Geometry: see drawing. Coordinates: mm, zero at the bounding-box minimum. Give positions to 0.01 mm unless a question says otherwise; leave off trailing zeros. Write each loop counter-clockwise with the first axis right and the second up, starting at its lowest first coordinate (ties: lowest second). Pieces come first, ordered by that corner, then holes. Notation, with made-up numbers: (49.25, 72.5) -> (95.25, 72.5) arc R24 cw to (95.25, 95.5) -> close; hole circle Ø1 at (-5.75, 73.5). An arc over 180 degrees is marked (long way). Answer as a JSON object with one key per item and string values. Group by question number.
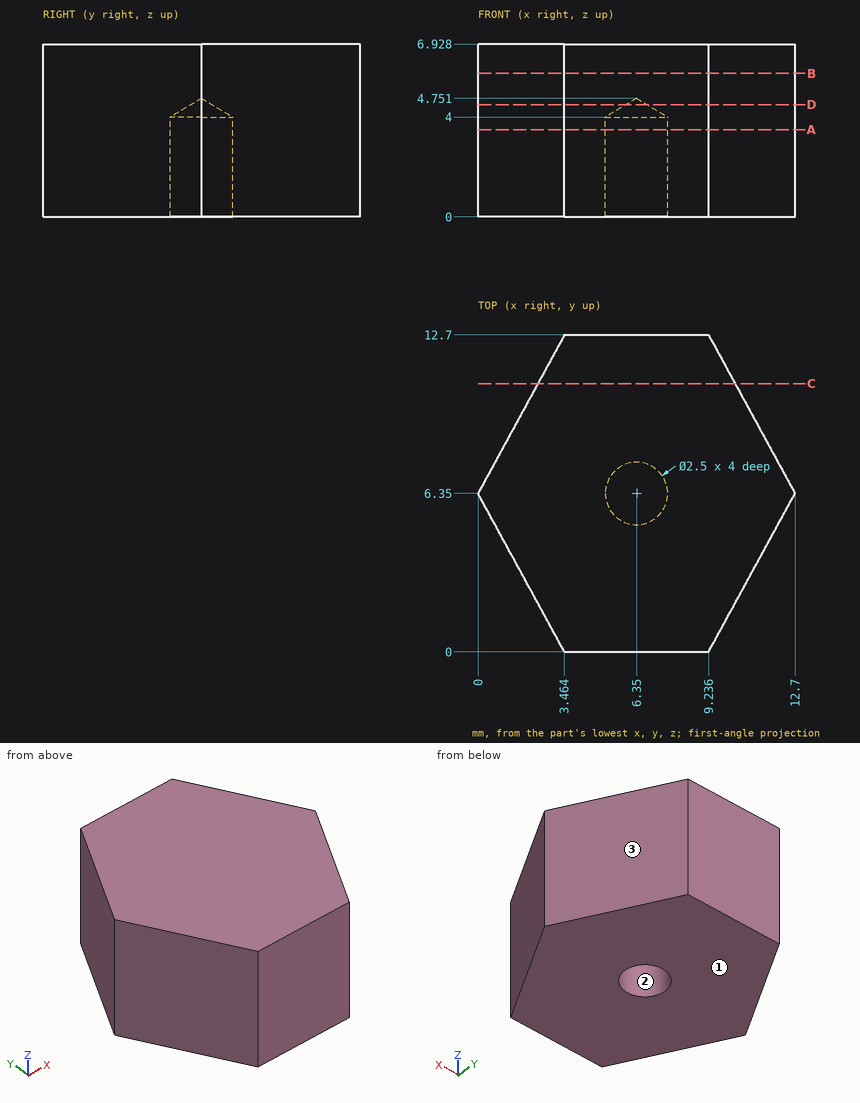
1. Section D-D (z = 4.5). Return the cut outline in (x, y), plus the area to 3 significant figures.
2. Line query: line 1 (Y direction, x = 6.35, z = 3.2); line 2 (Y direction, x = 5.75, z = 2); line 3 (X direction, y = 4.75, z = 4.75). Output: solid intervals per line, ascending.
3. Section B-B (z = 5.75). Return the cut outline in (x, y), plus the area to 3 significant figures.
4. Section A-A (z = 3.5). Return the cut outline in (x, y), plus the area to 3 significant figures.
5. Section C-C (y = 10.75). Return the cut outline in (x, z), plus the area to 3 significant figures.
6. Contact query for flat-ended pins moving along their axis: pin 1 Ø2 at (y, z) = (8, 4.5) entering from -X; pin 2 Ø2 at (x, y) = (6.35, 6.35) entering from -Z; pin 3 Ø2 at (y, z) = (2.5, 3) entering from +X. Output: stop coordinate, or through.
7. Mould query, pull axis X, two halves, no side actions, for the marked faces 1, 2 and 3. Classes: pulls with the +X half, pulls with the -X half, needs draft (parallel to the pull), parting line crosses it, or undercut.
Working result:
{
 "1": {"outline": "(0, 6.35) -> (3.46, 0) -> (9.24, 0) -> (12.7, 6.35) -> (9.24, 12.7) -> (3.46, 12.7) -> close; hole circle Ø0.84 at (6.35, 6.35)", "area": "117 mm^2"},
 "2": {"line 1": "y = 0 to 5.1, 7.6 to 12.7", "line 2": "y = 0 to 5.25, 7.45 to 12.7", "line 3": "x = 0.87 to 11.83"},
 "3": {"outline": "(0, 6.35) -> (3.46, 0) -> (9.24, 0) -> (12.7, 6.35) -> (9.24, 12.7) -> (3.46, 12.7) -> close", "area": "117 mm^2"},
 "4": {"outline": "(0, 6.35) -> (3.46, 0) -> (9.24, 0) -> (12.7, 6.35) -> (9.24, 12.7) -> (3.46, 12.7) -> close; hole circle Ø2.5 at (6.35, 6.35)", "area": "112 mm^2"},
 "5": {"outline": "(2.4, 0) -> (10.3, 0) -> (10.3, 6.93) -> (2.4, 6.93) -> close", "area": "54.7 mm^2"},
 "6": {"pin 1": "stops at x = 0.35", "pin 2": "stops at z = 4.15", "pin 3": "stops at x = 11.15"},
 "7": {"face 1": "needs draft", "face 2": "undercut", "face 3": "pulls with the +X half"}
}
